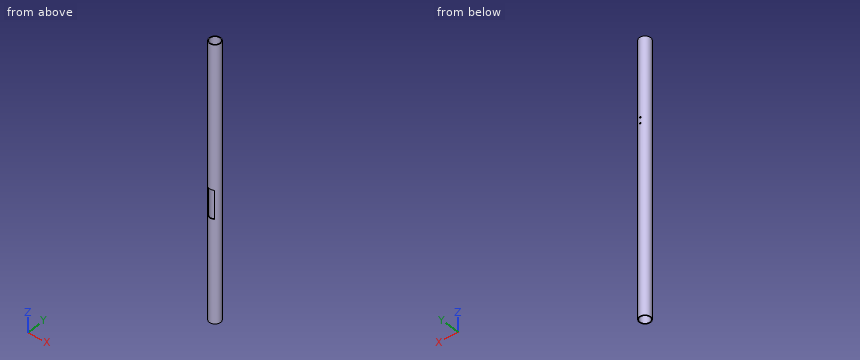
from build123d import *

# Parameters (mm, degrees)
SKETCH1_R               = 12.7
SKETCH1_R_2             = 11.049
BOSS_EXTRUDE1_DEPTH     = 609.6
SKETCH2_R               = 11.0998
SKETCH2_R_2             = 11.049
CUT_EXTRUDE1_DEPTH      = 76.2
CUT_EXTRUDE2_REACH      = 612.261
CUT_EXTRUDE2_END_RADIUS = 11.049
SKETCH5_R               = 1.651
CUT_EXTRUDE3_REACH      = 612.261
CUT_EXTRUDE3_END_RADIUS = 11.049
SKETCH6_W               = 15.24
SKETCH6_H               = 63.5


with BuildPart() as part:
    # Sketch1 → Boss-Extrude1 (new body)
    with BuildSketch(Plane.XY):
        with Locations(Location((0, 0, 0), (0, 0, 180))):
            Circle(SKETCH1_R)
        with Locations(Location((0, 0, 0), (0, 0, 180))):
            Circle(SKETCH1_R_2, mode=Mode.SUBTRACT)
    extrude(amount=BOSS_EXTRUDE1_DEPTH)

    # Sketch2 → Cut-Extrude1 (cut)
    with BuildSketch(Plane.XY):
        with Locations(Location((0, 0, 0), (0, 0, 180))):
            Circle(SKETCH2_R)
        with Locations(Location((0, 0, 0), (0, 0, 180))):
            Circle(SKETCH2_R_2, mode=Mode.SUBTRACT)
    extrude(amount=CUT_EXTRUDE1_DEPTH, mode=Mode.SUBTRACT)

    # Cut-Extrude2: up to this cylinder (the profile starts outside it)
    cut_extrude2_end = Plane(origin=(0, 0, 427.6725), z_dir=(0, 0, -1)) * Cylinder(CUT_EXTRUDE2_END_RADIUS, 1260.32, mode=Mode.PRIVATE)
    # Sketch5 → Cut-Extrude2 (cut, up to the surface)
    with BuildSketch(Plane(origin=(0, 12.7, 0), x_dir=(1, 0, 0), z_dir=(0, 1, 0)), mode=Mode.PRIVATE) as cut_extrude2_sk1:
        with Locations(Location((0, -434.0225, 0), (0, 0, 270))):
            Circle(SKETCH5_R)
    cut_extrude2_tool1 = extrude(cut_extrude2_sk1.sketch, amount=-CUT_EXTRUDE2_REACH, mode=Mode.PRIVATE) - cut_extrude2_end
    add(cut_extrude2_tool1.solids().sort_by_distance((0, 12.7, 434.0225))[0], mode=Mode.SUBTRACT)
    # Sketch5 → Cut-Extrude2 (cut, up to the surface)
    with BuildSketch(Plane(origin=(0, 12.7, 0), x_dir=(1, 0, 0), z_dir=(0, 1, 0)), mode=Mode.PRIVATE) as cut_extrude2_sk2:
        with Locations(Location((0, -421.3225, 0), (0, 0, 270))):
            Circle(SKETCH5_R)
    cut_extrude2_tool2 = extrude(cut_extrude2_sk2.sketch, amount=-CUT_EXTRUDE2_REACH, mode=Mode.PRIVATE) - cut_extrude2_end
    add(cut_extrude2_tool2.solids().sort_by_distance((0, 12.7, 421.3225))[0], mode=Mode.SUBTRACT)

    # Cut-Extrude3: up to this cylinder (the profile starts outside it)
    cut_extrude3_end = Plane(origin=(0, 0, 260.35), z_dir=(0, 0, -1)) * Cylinder(CUT_EXTRUDE3_END_RADIUS, 1247.62, mode=Mode.PRIVATE)
    # Sketch6 → Cut-Extrude3 (cut, up to the surface)
    with BuildSketch(Plane(origin=(0, -12.7, 0), x_dir=(-1, 0, 0), z_dir=(0, -1, 0)), mode=Mode.PRIVATE) as cut_extrude3_sk1:
        with Locations((0, -260.35)):
            Rectangle(SKETCH6_W, SKETCH6_H)
    cut_extrude3_tool1 = extrude(cut_extrude3_sk1.sketch, amount=-CUT_EXTRUDE3_REACH, mode=Mode.PRIVATE) - cut_extrude3_end
    add(cut_extrude3_tool1.solids().sort_by_distance((0, -12.7, 260.35))[0], mode=Mode.SUBTRACT)


solid = part.part
The listing builds one solid part. Answer for the finished solid, in the listing's coordinates (mm). Coordinates: 2 decimals unless noted, no trailing zeros. Order: outer loops, then holes, each group sorted by start corner. A loop starts at its lowest first (then second) coordinate and runs counter-clockwise, first axis right, second up. Notation, with made-up numbers: (-29.5, -14) -> (-1.5, -14) arc R6 cw to (-1.5, -7) -> close; hole circle Ø3 at (27.25, 31.5). An arc over 180 degrees is marked (long way). Answer in a Markdown table with one row per item. Add a question column.
Item 1: Find the intervals of material crossed by L1, parallel to Z at x = 0, y = 11.85; L2, parallel to Y at x = 0, z = 60; L3, parallel to X at y = -0.75, z = 394, in increasing order. Write a range as from..to.
Item 2: Find section B-B (z = 267.5). Write down the section's boundary in (x, y), then the cut area to 3 significant figures.
Item 3: Find section A-A (y = 0). Write down the section's boundary in (x, z), then the cut area to 3 significant figures.
Item 4: Each of these flat-tipped pins is pushed along its axis until it touches: P1, Ø13.5, axis at x = 0, y = 0, coming from the -Z side; P2, Ø3, axis at x = 3.5, z = 211.5, coming from the +Y side; P3, Ø0.6, axis at y = -9.5, z = 270, coming from the -X side (3 decimals); P4, Ø2.5, axis at y = -9, z = 275.5, coming from the +X side. Where does it stop, or does it pass through?
Result set:
| question | item | result |
|---|---|---|
| 1 | L1 | z = 0..419.67, 422.97..432.37, 435.67..609.6 |
| 1 | L2 | y = -12.7..-11.1, 11.1..12.7 |
| 1 | L3 | x = -12.68..-11.02, 11.02..12.68 |
| 2 | outline | (-7.62, -10.16) -> (-7.62, -8) arc R11.05 cw (long way) to (7.62, -8) -> (7.62, -10.16) arc R12.7 ccw (long way) to start |
| 2 | area | 95.8 mm² |
| 3 | outline | (-12.7, 0) -> (-11.1, 0) -> (-11.1, 76.2) -> (-11.05, 76.2) -> (-11.05, 609.6) -> (-12.7, 609.6) -> close; (11.05, 76.2) -> (11.1, 76.2) -> (11.1, 0) -> (12.7, 0) -> (12.7, 609.6) -> (11.05, 609.6) -> close |
| 3 | area | 2,010 mm² |
| 4 | P1 | passes through |
| 4 | P2 | stops at y = 12.54 |
| 4 | P3 | stops at x = -8.755 |
| 4 | P4 | stops at x = 10.06 |
